The model under review builds one solid part; all positions refer to its coordinate system, in mm. Coordinates: 2 decimals unless noted, no trailing zeros. Order: outer loops, then holes, each group sorted by start corner. A loop starts at its lowest first (then second) coordinate and runs counter-clockwise, first axis right, second up. Notation, with made-up numbers: M -27.75,-9.5 L 26.25,-9.5 A26 cw 26.25,21.5 Z; hole C 83,-18 d4. An arc over 180 degrees is marked long. Answer in a Markdown table with one row per item.
from build123d import *

# Parameters (mm, degrees)
SKETCH1_R        = 0.254
EXTRUDE1_DEPTH   = 2.54
EXTRUDE1_2_DEPTH = 2.54
EXTRUDE1_3_DEPTH = 2.54
EXTRUDE1_4_DEPTH = 2.54
EXTRUDE1_5_DEPTH = 2.54
EXTRUDE1_6_DEPTH = 2.54
SKETCH2_W        = 10.16
SKETCH2_H        = 18.8976
EXTRUDE2_DEPTH   = 7.62


with BuildPart() as part:
    # Sketch1 → Extrude1 (new body)
    with BuildSketch(Plane.XY):
        Circle(SKETCH1_R)
    extrude(amount=EXTRUDE1_DEPTH)



with BuildPart() as body_2:
    # Sketch1 → Extrude1 2 (new body)
    with BuildSketch(Plane.XY):
        with Locations((2.54, 0)):
            Circle(SKETCH1_R)
    extrude(amount=EXTRUDE1_2_DEPTH)


with BuildPart() as body_3:
    # Sketch1 → Extrude1 3 (new body)
    with BuildSketch(Plane.XY):
        with Locations((5.08, 0)):
            Circle(SKETCH1_R)
    extrude(amount=EXTRUDE1_3_DEPTH)


with BuildPart() as body_4:
    # Sketch1 → Extrude1 4 (new body)
    with BuildSketch(Plane.XY):
        with Locations((7.62, 0)):
            Circle(SKETCH1_R)
    extrude(amount=EXTRUDE1_4_DEPTH)


with BuildPart() as body_5:
    # Sketch1 → Extrude1 5 (new body)
    with BuildSketch(Plane.XY):
        with Locations((0, -7.62)):
            Circle(SKETCH1_R)
    extrude(amount=EXTRUDE1_5_DEPTH)


with BuildPart() as body_6:
    # Sketch1 → Extrude1 6 (new body)
    with BuildSketch(Plane.XY):
        with Locations((7.62, -7.62)):
            Circle(SKETCH1_R)
    extrude(amount=EXTRUDE1_6_DEPTH)


with BuildPart() as part_1:
    add(part.part)

    add(body_2.part)  # Extrude2 merges body 2

    add(body_3.part)  # Extrude2 merges body 3

    add(body_4.part)  # Extrude2 merges body 4

    add(body_5.part)  # Extrude2 merges body 5

    add(body_6.part)  # Extrude2 merges body 6
    # Sketch2 → Extrude2 (add)
    with BuildSketch(Plane(origin=(0, 0, 0), x_dir=(-1, 0, 0), z_dir=(0, 0, -1))):
        with Locations((-3.81, -6.4516)):
            Rectangle(SKETCH2_W, SKETCH2_H)
    extrude(amount=EXTRUDE2_DEPTH)


solid = part_1.part
(1) Take a section at D-D (y = 0). Write out the cut boundary in (x, z).
Report:
| item | result |
|---|---|
| outline | M -1.27,-7.62 L 8.89,-7.62 L 8.89,0 L 7.87,0 L 7.87,2.54 L 7.37,2.54 L 7.37,0 L 5.33,0 L 5.33,2.54 L 4.83,2.54 L 4.83,0 L 2.79,0 L 2.79,2.54 L 2.29,2.54 L 2.29,0 L 0.25,0 L 0.25,2.54 L -0.25,2.54 L -0.25,0 L -1.27,0 Z |
(2) To check wall thickness, follow line 1 (Z direction, x = 5.25, y = -1.75). State the ranges of the line that lie inside material, in increasing order. Write a range as [from, to].
Report:
| item | result |
|---|---|
| line 1 | [-7.62, 0] |
(3) Take a section at B-B (y = -7.62). Write out the cut boundary in (x, z), then the cut area to 3 significant figures.
Report:
| item | result |
|---|---|
| outline | M -1.27,-7.62 L 8.89,-7.62 L 8.89,0 L 7.87,0 L 7.87,2.54 L 7.37,2.54 L 7.37,0 L 0.25,0 L 0.25,2.54 L -0.25,2.54 L -0.25,0 L -1.27,0 Z |
| area | 80.0 mm^2 |
(4) Take a section at A-A (z = 0.5). Write out the cut boundary in (x, y), then the cut area to 3 significant figures.
Report:
| item | result |
|---|---|
| outline | C 0,-7.62 d0.51; C 0,0 d0.51; C 2.54,0 d0.51; C 5.08,0 d0.51; C 7.62,-7.62 d0.51; C 7.62,0 d0.51 |
| area | 1.22 mm^2 |
(5) Take a section at C-C (x = 7.62). Write out the cut boundary in (y, z).
Report:
| item | result |
|---|---|
| outline | M -15.9,-7.62 L 3,-7.62 L 3,0 L 0.25,0 L 0.25,2.54 L -0.25,2.54 L -0.25,0 L -7.37,0 L -7.37,2.54 L -7.87,2.54 L -7.87,0 L -15.9,0 Z |
